from build123d import *

# Parameters (mm, degrees)
SKETCH_6_R                 = 72.75
EXTRUDE_16_DEPTH           = 100
SHELL_8_T                  = -10
CUT_EXTRUDE_START          = -40
SKETCH_13_R                = 68.75
SKETCH_13_R_2              = 62.75
CUT_EXTRUDE_5_DEPTH        = 40
F_16_0MM_2_REACH           = 180.442
F_16_0MM_2_BORE_R          = 8
F_16_0MM_2_ON_FACE_2_REACH = 185.929
F_16_0MM_2_BORE_2_R        = 8


with BuildPart() as part:
    # 草圖6 → 填料-伸長16 (new body)
    with BuildSketch(Plane(origin=(0, 0, 0), x_dir=(1, 0, 0), z_dir=(0, 1, 0))):
        with Locations(Location((0, 0, 0), (0, 0, 270))):
            Circle(SKETCH_6_R)
    extrude(amount=EXTRUDE_16_DEPTH)

    # 薄殼8
    shell_8_openings = [part.faces().sort_by_distance(p)[0] for p in [
        (0, 100, 0),
    ]]
    offset(amount=SHELL_8_T, openings=shell_8_openings, kind=Kind.INTERSECTION)

    # 草圖13 → 除料-伸長5 (cut)
    with BuildSketch(Plane(origin=(0, 100, 0), x_dir=(1, 0, 0), z_dir=(0, 1, 0)).offset(CUT_EXTRUDE_START)):
        with Locations(Location((0, 0, 0), (0, 0, 270))):
            Circle(SKETCH_13_R)
        with Locations(Location((0, 0, 0), (0, 0, 270))):
            Circle(SKETCH_13_R_2, mode=Mode.SUBTRACT)
    extrude(amount=CUT_EXTRUDE_5_DEPTH, mode=Mode.SUBTRACT)

    # Ø16.0mm 定位孔2 bore (on position points) → Ø16.0mm 定位孔2 (cut, up to next)
    with BuildSketch(Plane(origin=(7.281311378, 33.875955165, 72.384701454), x_dir=(0.994978714148, 0, -0.100086754332), z_dir=(0.100086754332, 0, 0.994978714148)), mode=Mode.PRIVATE) as f_16_0mm_2_sk1:
        Circle(F_16_0MM_2_BORE_R)
    f_16_0mm_2_tool1 = extrude(f_16_0mm_2_sk1.sketch, amount=-F_16_0MM_2_REACH, mode=Mode.PRIVATE) & part.part
    add(f_16_0mm_2_tool1.solids().sort_by_distance((7.281311, 33.875955, 72.384701))[0], mode=Mode.SUBTRACT)

    # Ø16.0mm 定位孔2 bore 2 (on position points) → Ø16.0mm 定位孔2 on face 2 (cut, up to next)
    with BuildSketch(Plane(origin=(7.98509872, 79.17918137, 72.310446676), x_dir=(0.993958008506, 0, -0.109761000939), z_dir=(0.109761000939, 0, 0.993958008506)), mode=Mode.PRIVATE) as f_16_0mm_2_on_face_2_sk1:
        Circle(F_16_0MM_2_BORE_2_R)
    f_16_0mm_2_on_face_2_tool1 = extrude(f_16_0mm_2_on_face_2_sk1.sketch, amount=-F_16_0MM_2_ON_FACE_2_REACH, mode=Mode.PRIVATE) & part.part
    add(f_16_0mm_2_on_face_2_tool1.solids().sort_by_distance((7.985099, 79.179181, 72.310447))[0], mode=Mode.SUBTRACT)


solid = part.part
For this review, take the finished solid that the model builds, in its own axes (mm). A direction names the side the tool comes from. Coordinates: 2 decimals unless noted, no trailing zeros. Order: outer loops, then holes, each group sorted by start corner. A loop starts at its lowest first (then second) coordinate and runs counter-clockwise, first axis right, second up. Notation, with made-up numbers: (-23, 3.5) -> (17, 3.5) arc R4 ccw to (17, 8.5) -> close; hole circle Ø8 at (57, 60). An arc over 180 degrees is marked (long way). Return JSON: item names as keys, results as strings.
1. We need section A-A on z = 0. Write out the cut boundary in (x, y).
Answer block:
{"outline": "(-72.75, 0) -> (72.75, 0) -> (72.75, 100) -> (68.75, 100) -> (68.75, 60) -> (62.75, 60) -> (62.75, 10) -> (-62.75, 10) -> (-62.75, 60) -> (-68.75, 60) -> (-68.75, 100) -> (-72.75, 100) -> close"}
2. We need section C-C on x = 31.5. Write out the cut boundary in (y, z).
Answer block:
{"outline": "(0, -65.58) -> (100, -65.58) -> (100, -61.11) -> (60, -61.11) -> (60, -54.27) -> (10, -54.27) -> (10, 54.27) -> (60, 54.27) -> (60, 61.11) -> (100, 61.11) -> (100, 65.58) -> (0, 65.58) -> close"}
3. Machinability: for faces 1 (the cylindrical face through (42.41, 34.65, -46.25)), 2 (the cylindrical face through (5.037, 26.066, 67.402)), which of the approach directions +Z, -Z, +X, -X, +Y, -Y give a long, thin tool a straight path to every point of the face, cutting with its end or side? Answer none if there is none.
Answer block:
{"face 1": "+Y", "face 2": "none"}
4. For pin 1 Ø12 at (y, z) = (54.5, -34.5) entering from -X; pin 2 Ø10 at (x, y) = (28, 59.5) entering from -Z; pin 3 Ø1 at (x, y) = (-45.5, 14.5) entering from +Z, all flat-tipped, find the tip position at first contact; note any pin that passes through.
Answer block:
{"pin 1": "x = -66.94", "pin 2": "z = -69.02", "pin 3": "z = 57.16"}
5. The part is to be moulded in two halves that separate along Z. For faces 3 (the flat face through (43, 100, 54)), 4 (the cylindrical face through (6.02, 71.37, 70.31)), 5 (the cylindrical face through (-44.27, 49.3, -57.73)), say which applies: +Z half, -Z half, draft (parallel to the pull), parting line (faces both ways), or undercut.
Answer block:
{"face 3": "draft", "face 4": "undercut", "face 5": "parting line"}
6. For line 1 (X direction, y = 39.5, z = 0); line 2 (Y direction, x = -28, z = -16.5); line 3 (Z direction, x = 56, y = 71), list the stretches that pass through material, from the lowest coordinate up. Write a range as from..to.
Answer block:
{"line 1": "-72.75..-62.75, 62.75..72.75", "line 2": "0..10", "line 3": "-46.44..-39.88, 39.88..46.44"}
7. We need section B-B on y = 20. Write out the cut boundary in (x, z), and give its area (3 significant figures).
Answer block:
{"outline": "circle Ø145.5 at (0, 0); hole circle Ø125.5 at (0, 0)", "area": "4,260 mm²"}
